Autodesk Inventor part; units mm, degrees
ref_plane "YZ Plane" through (0, 0, 0) normal (1, 0, 0) x (0, 1, 0)
ref_plane "XZ Plane" through (0, 0, 0) normal (0, 1, 0) x (-1, 0, 0)
ref_plane "XY Plane" through (0, 0, 0) normal (0, 0, 1) x (1, 0, 0)
ref_plane "Work Plane1" through (0, 0, 0) normal (0, 0, -1) x (-1, 0, 0)
sketch "Sketch1" plane through (0, 0, 0) normal (0, 0, -1) x (-1, 0, 0)
  line L0 (-115.3126, -90.0255) -> (64.6874, -90.0255)
  line L1 (64.6874, -90.0255) -> (64.6874, 89.9745)
  line L2 (64.6874, 89.9745) -> (-115.3126, 89.9745)
  line L3 (-115.3126, 89.9745) -> (-115.3126, -90.0255)
  line L4 (-25.3126, 0) -> (-25.3126, -88.1346) construction
  line L5 (-1.4905, -0.0255) -> (99.3864, -0.0255) construction
  point P0 (0, 0)
  point P1 (-25.3126, -0.0255)
  dimension "d0" = 180
  dimension "d1" = 180
  dimension "d8" = 90
  dimension "d9" = 90
extrude "Extrusion1" add sketch "Sketch1" along normal mid plane 2
sketch "Sketch2" plane through (0, 0, -1) normal (0, 0, -1) x (-1, 0, 0)
  circle A0 centre (-25, 0) radius 25.15
  point P0 (0, 0)
extrude "Extrusion2" cut sketch "Sketch2" against normal through all
ref_plane "Work Plane3" through (0, 0, -56) normal (0, 0, -1) x (-1, 0, 0)
ref_plane "Work Plane2" through (0, 0, -116) normal (0, 0, -1) x (-1, 0, 0)
equation "\"d1\" = d0"
properties part number "tapa_dummy"
The listing builds one solid part. Answer for the finished solid, in the listing's coordinates (mm). Give positions to 0.01 mm unless a question says otherwise; leave off trailing zeros. Loops run counter-clockwise (first coordinate to the right, second up) from the corner with the lowest first, then second, coordinate; pieces in that order, holes last. Notation, with made-up numbers: (42, 58) - (65, 58) arc R34 cw to (65, 92) - close; hole circle Ø7 at (88, -21.75). An arc over 180 degrees is marked (long way). Answer as CSV lines item,"result". Start each with the question number.
Item 1: Find the intervals of material crossed by line 1 (Y direction, x = 25, z = 0.6); line 2 (X direction, y = 5.5, z = -0.2); line 3 (X direction, y = -9, z = 0.3), in increasing order. Write a range as from..to.
Item 2: The mould has two halves that part along X. Classify faces 1 (the face through (28.274, 24.936, -0.014)), 2 (the face through (7, 21, -1)): +X half, -X half, draft (parallel to the pull), parting line (faces both ways), or undercut.
Item 3: A cutting plane is placed at B-B on y = 0. Determine the outline of the cut face in (x, z).
Item 4: A cutting plane is placed at A-A on x = 25. Determine the outline of the cut face in (y, z), then the cut area to 3 significant figures.
Item 5: A cutting plane is placed at C-C on z = 0.65. Determine the outline of the cut face in (x, y).
Found:
1,line 1,"y = -90.03..-25.15, 25.15..89.97"
1,line 2,"x = -64.69..0.46, 49.54..115.31"
1,line 3,"x = -64.69..1.52, 48.48..115.31"
2,face 1,"undercut"
2,face 2,"draft"
3,outline,"(-64.69, -1) - (-0.15, -1) - (-0.15, 1) - (-64.69, 1) - close; (50.15, -1) - (115.31, -1) - (115.31, 1) - (50.15, 1) - close"
4,outline,"(-90.03, -1) - (-25.15, -1) - (-25.15, 1) - (-90.03, 1) - close; (25.15, -1) - (89.97, -1) - (89.97, 1) - (25.15, 1) - close"
4,area,"259 mm^2"
5,outline,"(-64.69, -90.03) - (115.31, -90.03) - (115.31, 89.97) - (-64.69, 89.97) - close; hole circle Ø50.3 at (25, 0)"
